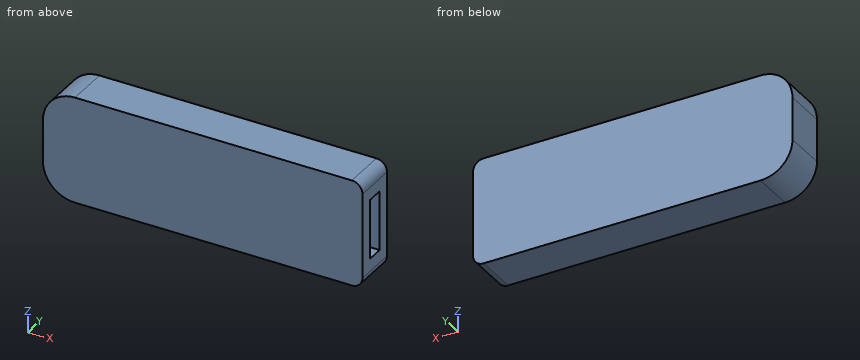
from build123d import *

# Parameters (mm, degrees)
SKETCH1_W           = 30
SKETCH1_H           = 10
BOSS_EXTRUDE1_DEPTH = 4
SKETCH2_W           = 5.6
SKETCH2_H           = 1.6
CUT_EXTRUDE1_DEPTH  = 13
FILLET1_R           = 3
FILLET2_R           = 1


with BuildPart() as part:
    # Sketch1 → Boss-Extrude1 (new body)
    with BuildSketch(Plane(origin=(0, 0, 0), x_dir=(1, 0, 0), z_dir=(0, 1, 0))):
        with Locations((-15, 5)):
            Rectangle(SKETCH1_W, SKETCH1_H)
    extrude(amount=BOSS_EXTRUDE1_DEPTH)

    # Sketch2 → Cut-Extrude1 (cut)
    with BuildSketch(Plane(origin=(0, 0, 0), x_dir=(0, 0, -1), z_dir=(1, 0, 0))):
        with Locations((5, 2)):
            Rectangle(SKETCH2_W, SKETCH2_H)
    extrude(amount=-CUT_EXTRUDE1_DEPTH, mode=Mode.SUBTRACT)

    # Fillet1
    fillet1_edges = [part.edges().sort_by_distance(p)[0] for p in [
        (-30, 2, 0),
        (-30, 2, -10),
    ]]
    fillet(fillet1_edges, radius=FILLET1_R)

    # Fillet2
    fillet2_edges = [part.edges().sort_by_distance(p)[0] for p in [
        (0, 2, 0),
        (0, 2, -10),
    ]]
    fillet(fillet2_edges, radius=FILLET2_R)


solid = part.part
The listing builds one solid part. Answer for the finished solid, in the listing's coordinates (mm). Give positions to 0.01 mm unless a question says otherwise; leave off trailing zeros. Loops run counter-clockwise (first coordinate to the right, second up) from the corner with the lowest first, then second, coordinate; pieces in that order, holes last.
Item 1: A cutting plane is placed at C-C (y = 2.15). Give the vertices of the cut face in (x, z).
Derived:
outline: (-30, -7) arc R3 ccw to (-27, -10) - (-1, -10) arc R1 ccw to (0, -9) - (0, -7.8) - (-13, -7.8) - (-13, -2.2) - (0, -2.2) - (0, -1) arc R1 ccw to (-1, 0) - (-27, 0) arc R3 ccw to (-30, -3) - close
Item 2: A cutting plane is placed at A-A (x = -5.5). Give the vertices of the cut face in (y, z), then the cut area to 3 significant figures.
Derived:
outline: (0, -10) - (4, -10) - (4, 0) - (0, 0) - close; hole (1.2, -7.8) - (2.8, -7.8) - (2.8, -2.2) - (1.2, -2.2) - close
area: 31.0 mm2
Item 3: Find the intervals of material crossed by line 1 along Y through (x, z) = (-4, -4.5); line 2 along Z through (x, y) = (-9.5, 2.6); line 3 along X through (y, z) = (1.35, -3.25), in increasing order.
Derived:
line 1: y = 0 to 1.2, 2.8 to 4
line 2: z = -10 to -7.8, -2.2 to 0
line 3: x = -30 to -13
Item 4: A cutting plane is placed at B-B (z = -4). Give the vertices of the cut face in (x, y).
Derived:
outline: (-30, 0) - (0, 0) - (0, 1.2) - (-13, 1.2) - (-13, 2.8) - (0, 2.8) - (0, 4) - (-30, 4) - close
